```python
from build123d import *

# Parameters (mm, degrees)
EXTRUDE_1_DEPTH      = 4
SKETCH_2_R           = 2.4
CUT_EXTRUDE_1_DEPTH  = 4
EXTRUDE_3_DEPTH      = 3
CUT_EXTRUDE_2_DEPTH  = 1
SKETCH_7_R           = 10.8
CUT_EXTRUDE_4_DEPTH  = 4
SKETCH_8_R           = 11.8
SKETCH_8_R_2         = 10.8
EXTRUDE_4_DEPTH      = 16.5
SKETCH_9_R           = 10.8
SKETCH_9_R_2         = 6.05
EXTRUDE_5_DEPTH      = 3.5
CUT_EXTRUDE_5_DEPTH  = 2.5
SKETCH_13_W          = 9
SKETCH_13_H          = 5
EXTRUDE_7_DEPTH      = 8.5
SKETCH_16_R          = 1.4
CUT_EXTRUDE_8_DEPTH  = 10
SKETCH_19_ONE_SIDE_W = 4.5
SKETCH_19_ONE_SIDE_H = 5
SKETCH_20_R          = 1.75
CUT_EXTRUDE_9_DEPTH  = 36.75966317


with BuildPart() as part:
    # Sketch 1 → Extrude 1 (new body)
    with BuildSketch(Plane(origin=(0, 0, 0), x_dir=(1, 0, 0), z_dir=(0, 1, 0))):
        Polygon((13.776603565, -33.25966317), (33.25966317, -13.776603565), (33.25966317, 13.776603565), (13.776603565, 33.25966317), (-13.776603565, 33.25966317), (-33.25966317, 13.776603565), (-33.25966317, -13.776603565), (-13.776603565, -33.25966317), align=None)
    extrude(amount=EXTRUDE_1_DEPTH)

    # Sketch 2 → Cut-Extrude 1 (cut)
    with BuildSketch(Plane.XZ):
        with Locations((0, -25)):
            Circle(SKETCH_2_R)
    extrude(amount=-CUT_EXTRUDE_1_DEPTH, mode=Mode.SUBTRACT)

    # Sketch 3 → Extrude 3 (add)
    with BuildSketch(Plane(origin=(0, 4, 0), x_dir=(1, 0, 0), z_dir=(0, 1, 0))):
        Polygon((-13.776603565, 33.25966317), (-33.25966317, 13.776603565), (-33.25966317, -13.776603565), (-13.776603565, -33.25966317), (13.776603565, -33.25966317), (33.25966317, -13.776603565), (33.25966317, 13.776603565), (13.776603565, 33.25966317), align=None)
        Polygon((-12.285434741, 29.65966317), (-29.65966317, 12.285434741), (-29.65966317, -12.285434741), (-12.285434741, -29.65966317), (12.285434741, -29.65966317), (29.65966317, -12.285434741), (29.65966317, 12.285434741), (12.285434741, 29.65966317), align=None, mode=Mode.SUBTRACT)
    extrude(amount=EXTRUDE_3_DEPTH)

    # Sketch 5 → Cut-Extrude 2 (cut)
    with BuildSketch(Plane(origin=(0, 7, 0), x_dir=(1, 0, 0), z_dir=(0, 1, 0))):
        Polygon((32.05966317, -13.27954729), (32.05966317, 13.27954729), (13.27954729, 32.05966317), (-13.27954729, 32.05966317), (-32.05966317, 13.27954729), (-32.05966317, -13.27954729), (-13.27954729, -32.05966317), (13.27954729, -32.05966317), align=None)
        Polygon((30.85966317, 12.782491015), (12.782491015, 30.85966317), (-12.782491015, 30.85966317), (-30.85966317, 12.782491015), (-30.85966317, -12.782491015), (-12.782491015, -30.85966317), (12.782491015, -30.85966317), (30.85966317, -12.782491015), align=None, mode=Mode.SUBTRACT)
    extrude(amount=-CUT_EXTRUDE_2_DEPTH, mode=Mode.SUBTRACT)

    # Sketch 7 → Cut-Extrude 4 (cut)
    with BuildSketch(Plane.XZ):
        Circle(SKETCH_7_R)
    extrude(amount=-CUT_EXTRUDE_4_DEPTH, mode=Mode.SUBTRACT)

    # Sketch 8 → Extrude 4 (add)
    with BuildSketch(Plane.XZ):
        Circle(SKETCH_8_R)
        Circle(SKETCH_8_R_2, mode=Mode.SUBTRACT)
    extrude(amount=EXTRUDE_4_DEPTH)



with BuildPart() as body_2:
    # Sketch 9 → Extrude 5 (new body)
    with BuildSketch(Plane.XZ.offset(16.5)):
        Circle(SKETCH_9_R)
        Circle(SKETCH_9_R_2, mode=Mode.SUBTRACT)
    extrude(amount=EXTRUDE_5_DEPTH)


with BuildPart() as part_1:
    add(part.part)

    add(body_2.part)  # Revolve 1 merges body 2
    # Sketch 10 → Revolve 1 (revolve)
    with BuildSketch(Plane.XY):
        Polygon((-11.8, -16.5), (-10.8, -20), (-10.8, -16.5), align=None)
    revolve(axis=Axis((0, -20, 0), (0, 1, 0)))

    # Sketch 11 → Cut-Extrude 5 (cut)
    with BuildSketch(Plane(origin=(0, 4, 0), x_dir=(1, 0, 0), z_dir=(0, 1, 0))):
        with BuildLine():
            Line((-14, 8.65), (14.4, 8.65))
            ThreePointArc((14.4, 8.65), (23.05, 0), (14.4, -8.65))
            Line((14.4, -8.65), (-14, -8.65))
            ThreePointArc((-14, -8.65), (-22.65, 0), (-14, 8.65))
        make_face()
    extrude(amount=-CUT_EXTRUDE_5_DEPTH, mode=Mode.SUBTRACT)

    # Sketch 13 → Extrude 7 (add)
    with BuildSketch(Plane.XZ):
        with Locations((-28.75966317, 0)):
            Rectangle(SKETCH_13_W, SKETCH_13_H)
    extrude_7 = extrude(amount=EXTRUDE_7_DEPTH)

    # Sketch 16 → Cut-Extrude 8 (cut)
    with BuildSketch(Plane(origin=(0, 1.5, 0), x_dir=(1, 0, 0), z_dir=(0, 1, 0))):
        with Locations((-21, 0)):
            Circle(SKETCH_16_R)
    cut_extrude_8 = extrude(amount=-CUT_EXTRUDE_8_DEPTH, mode=Mode.SUBTRACT)

    # Mirror 2: Cut-Extrude 8 across plane
    add(cut_extrude_8.mirror(Plane(origin=(0, 0, 0), x_dir=(0, 0, 1), z_dir=(1, 0, 0))), mode=Mode.SUBTRACT)

    # Sketch 19 one side → Revolve 2 (revolve)
    with BuildSketch(Plane.XZ.offset(8.5)):
        with Locations((-26.50966317, 0)):
            Rectangle(SKETCH_19_ONE_SIDE_W, SKETCH_19_ONE_SIDE_H)
    revolve_2 = revolve(axis=Axis((-28.75966317, -8.5, 5.440491611), (0, 0, -1)))

    # Sketch 20 → Cut-Extrude 9 (cut, through all)
    with BuildSketch(Plane(origin=(0, 0, -2.5), x_dir=(-1, 0, 0), z_dir=(0, 0, -1))):
        with Locations((28.75966317, -8.5)):
            Circle(SKETCH_20_R)
    cut_extrude_9 = extrude(amount=-CUT_EXTRUDE_9_DEPTH, mode=Mode.SUBTRACT)

    # Mirror 3: Extrude 7, Revolve 2, Cut-Extrude 9 across plane
    add(extrude_7.mirror(Plane(origin=(0, 0, 0), x_dir=(0, 0, 1), z_dir=(1, 0, 0))))
    add(revolve_2.mirror(Plane(origin=(0, 0, 0), x_dir=(0, 0, 1), z_dir=(1, 0, 0))))
    add(cut_extrude_9.mirror(Plane(origin=(0, 0, 0), x_dir=(0, 0, 1), z_dir=(1, 0, 0))), mode=Mode.SUBTRACT)


solid = part_1.part
```
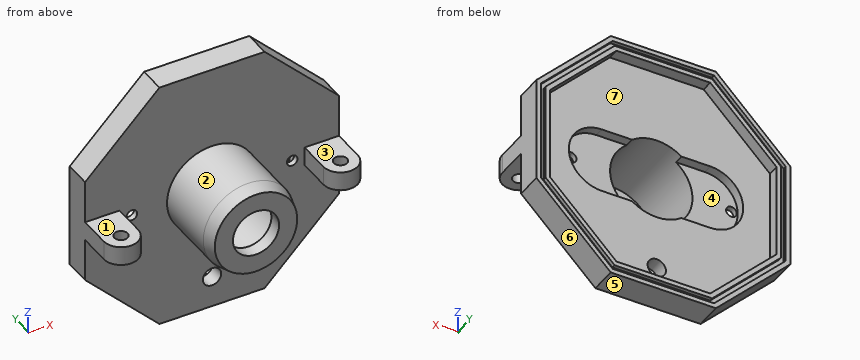
Model file for the job. Use its own axes, mm. Face numbers are marked on the shaded views. A direction names the side the tool comes from. Coordinates: 2 decimals unless noted, no trailing zeros. Loops run counter-clockwise (first coordinate to the right, second up) from the corner with the lowest first, then second, coordinate; pieces in that order, holes last. Notation, with made-up numbers: (43, 71) - (91, 71) arc R20 cw to (91, 100) - close; hole circle Ø10 at (-31, -20.5). An arc over 180 degrees is marked (long way). Answer as a JSON object with one key per item and string values. Group by question number.
(1) Probe line 1 along Z through (x, y) = (0, 1.7); line 2 along X through (y, z) = (-5.5, 0.5); line 3 along Z through (x, y) = (0, -6). List the from-to ranges inside material, lowest first.
(2) Cut at D-D (y = -14). Give the cut face in (x, z).
(3) Flat gauge pins, fed straight in: pin 1 (12 mm diameter, centred on x = 24, y = 1.5, fed in from +Z); pin 2 (5.5 mm diameter, centred on x = 28.76, y = -8.5, fed in from -Z); pin 3 (1.5 mm diameter, centred on x = -9.5, y = -8, fed in from -Z). Where does each tip first touch, or does it go through?
(4) Two-plate mould, pull along X, no slides. Class the marked faces 5, 6 and 7: released by +X, released by -X, zero draft, split by the parting line, or undercut.
(5) Cut at B-B (x = 21). Give the cut face in (y, z).
(6) Cut at A-A (z = -25). Give the cut face in (x, y), then the cut area to 3 significant figures.
(7) Cut at C-C (z = 0). State how many separate pieces and enclosed holes the cut face has, then the cut area to 3 significant figures.
(8) Tool access for the marked faces 1, 2, 3 and 4: list every direction of +Z, -Z, +X, -X, +Y, -Y with a clear straight run to the whole face (end or side of a thin tool).
Geometry says:
{
 "1": {"line 1": "z = -33.26 to -27.4, -22.6 to -10.8, 10.8 to 33.26", "line 2": "x = -33.26 to -24.26, -11.79 to -10.79, 10.79 to 11.79, 24.26 to 33.26", "line 3": "z = -11.8 to -10.8, 10.8 to 11.8"},
 "2": {"outline": "circle Ø23.6 at (0, 0); hole circle Ø21.6 at (0, 0)"},
 "3": {"pin 1": "stops at z = 29.04", "pin 2": "stops at z = -2.5", "pin 3": "stops at z = -7.92"},
 "4": {"face 5": "zero draft", "face 6": "released by +X", "face 7": "undercut"},
 "5": {"outline": "(0, -26.04) - (7, -26.04) - (7, -24.34) - (6, -24.34) - (6, -22.64) - (7, -22.64) - (7, -20.95) - (4, -20.95) - (4, -5.59) - (1.5, -5.59) - (1.5, -1.4) - (0, -1.4) - close; (0, 1.4) - (1.5, 1.4) - (1.5, 5.59) - (4, 5.59) - (4, 20.95) - (7, 20.95) - (7, 22.64) - (6, 22.64) - (6, 24.34) - (7, 24.34) - (7, 26.04) - (0, 26.04) - close"},
 "6": {"outline": "(-22.04, 0) - (-2.4, 0) - (-2.4, 4) - (-16.95, 4) - (-16.95, 7) - (-18.64, 7) - (-18.64, 6) - (-20.34, 6) - (-20.34, 7) - (-22.04, 7) - close; (2.4, 0) - (22.04, 0) - (22.04, 7) - (20.34, 7) - (20.34, 6) - (18.64, 6) - (18.64, 7) - (16.95, 7) - (16.95, 4) - (2.4, 4) - close", "area": "184 mm^2"},
 "7": {"separate pieces": "4", "enclosed holes": "2", "area": "397 mm^2"},
 "8": {"face 1": "+Z, -X, -Y", "face 2": "-Y", "face 3": "+Z, +X, -Y", "face 4": "+Y"}
}
